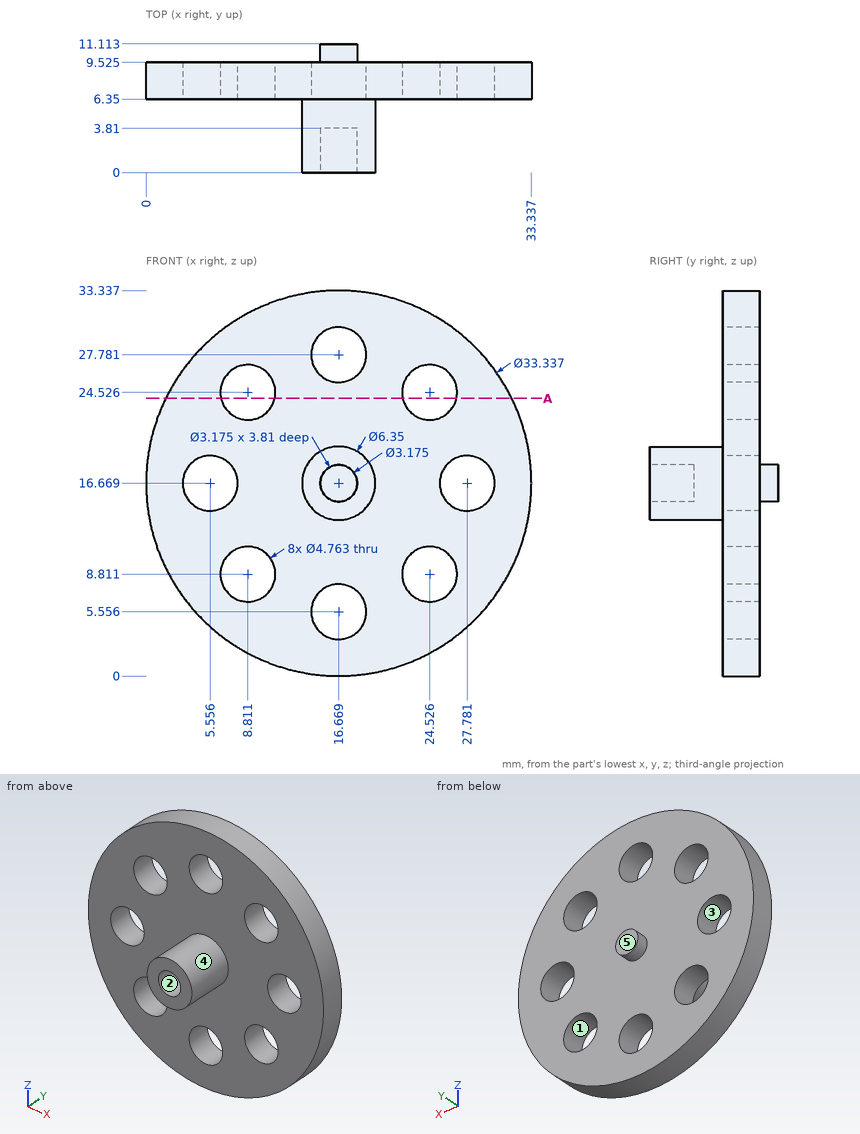
The drawing under review shows one solid part. Ordinate dimensions are in mm from its lowest x, y, z. A direction names the side the tool comes from. Round coordinates to 2 decimals unless told otherwise and drop trailing zeros. One line per question, with ' | ' between items.
(1) Take a section at A-A, the plane z = 24. State how many separate pieces and enclosed holes the cut face has.
Result sheet:
separate pieces: 3 | enclosed holes: 0
(2) Insertion check: P1, Ø3, axis at x = 27.78, z = 16.67, coming from the -Y side; P2, Ø6, axis at x = 16.67, z = 27.78, coming from the +Y side (1 decimal); P3, Ø1.6, axis at x = 16.5, z = 16, coming from the -Y side; P4, Ø6, axis at y = 6.5, z = 26, coming from the +X side. Each pin has a flat end and moves straight along its axis. Give the tip position at first contact, or say it passes through.
Result sheet:
P1: through | P2: y = 9.5 | P3: y = 3.81 | P4: x = 32.09
(3) Draft analysis for pull direction Z (two halves, no side actions). For the marked faces 3, 4 and 5, state which applies: released by +Z, released by -Z, zero draft, split by the parting line, or undercut.
Result sheet:
face 3: undercut | face 4: split by the parting line | face 5: zero draft
(4) Wall thickness on line 1 (X direction, y = 8.25, z = 9.5) (1 decimal); line 2 (Y direction, x = 17.5, z = 17); line 3 (Z direction, x = 28, y = 7.25) (1 decimal): over which ranges is each line inside the solid? List them lowest first. Write a range as [from, to].
Result sheet:
line 1: [1.6, 6.5], [11.1, 22.2], [26.8, 31.7] | line 2: [3.81, 11.11] | line 3: [4.4, 14.3], [19, 28.9]
(5) Machinability: for the marked faces 1 and 2, which of the approach directions +Z, -Z, +X, -X, +Y, -Y give a long, thin tool a straight path to every point of the face, cutting with its end or side? Answer none if there is none.
Result sheet:
face 1: +Y, -Y | face 2: -Y
